Verification items for this drawing (mm, ordinates from the low corner). A direction names the side the tool comes from. Coordinates: 2 decimals unless noted, no trailing zeros. Loops run counter-clockwise (first coordinate to the right, second up) from the corner with the lowest first, then second, coordinate; pieces in that order, holes last. Notation, with made-up numbers: M 15,37 L 38,37 A23 cw 38,45 Z; hole C -32.5,-27.75 d10. An arc over 180 degrees is marked long. Write each question's results on one line, items separated by ' | '. Start each with the question number.
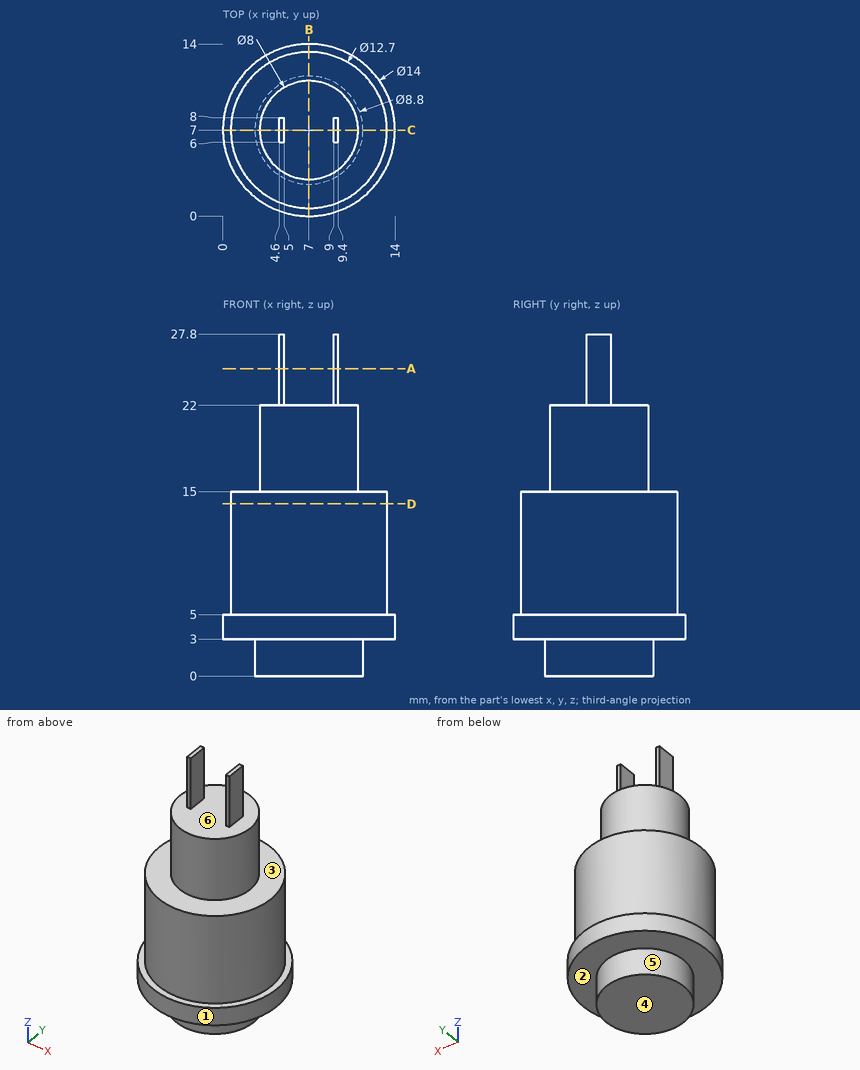
Item 1: Section check C-C (y = 7). Record the cut outline in (x, z).
Item 2: Release check for a two-part mould opening along X. For the marked faces 4, 5 and 6 record: +X half, -X half, draft (parallel to the pull), parting line (faces both ways), or undercut.
Item 3: Thickness scan on line 1 (X direction, y = 7, z = 22.5); line 2 (Z direction, x = 4.25, y = 6); line 3 (Z direction, x = 11.5, y = 5.75). Record the ranges inside material, lowest first.
Item 4: Section check D-D (z = 14). Record the cut outline in (x, y), plus the area to 3 significant figures.
Item 5: Section check B-B (x = 7). Record the cut outline in (y, z), plus the area to 3 significant figures.
Item 6: Tool access check on the marked faces 1, 2 and 3. Record the directions out of +Z, -Z, +X, -X, +Y, -Y that give a thin tool (end or side, any length) a straight path to the whole face; none if there is none.
Item 7: Depth check by flat-ended pin: P1, Ø1.5, axis at y = 8, z = 17.5, coming from the +X side; P2, Ø1, axis at y = 9.5, z = 14, coming from the -X side; P3, Ø1, axis at x = 1.5, y = 7, coming from the -Z side. Enter the tip coordinate at first touch or a pass-through.
Item 8: Section check A-A (z = 25). Record the cut outline in (x, y), plus the area to 3 significant figures.
Computed values:
1) outline: M 0,3 L 2.6,3 L 2.6,0 L 11.4,0 L 11.4,3 L 14,3 L 14,5 L 13.35,5 L 13.35,15 L 11,15 L 11,22 L 9.4,22 L 9.4,27.8 L 9,27.8 L 9,22 L 5,22 L 5,27.8 L 4.6,27.8 L 4.6,22 L 3,22 L 3,15 L 0.65,15 L 0.65,5 L 0,5 Z
2) face 4: draft | face 5: parting line | face 6: undercut
3) line 1: x = 4.6 to 5, 9 to 9.4 | line 2: z = 0 to 22 | line 3: z = 3 to 15
4) outline: C 7,7 d12.7 | area: 127 mm²
5) outline: M 0,3 L 2.6,3 L 2.6,0 L 11.4,0 L 11.4,3 L 14,3 L 14,5 L 13.35,5 L 13.35,15 L 11,15 L 11,22 L 3,22 L 3,15 L 0.65,15 L 0.65,5 L 0,5 Z | area: 237 mm²
6) face 1: +Z, -Z | face 2: -Z | face 3: +Z
7) P1: stops at x = 10.99 | P2: stops at x = 0.97 | P3: stops at z = 3
8) outline: M 4.6,6 L 5,6 L 5,8 L 4.6,8 Z; M 9,6 L 9.4,6 L 9.4,8 L 9,8 Z | area: 1.60 mm²
